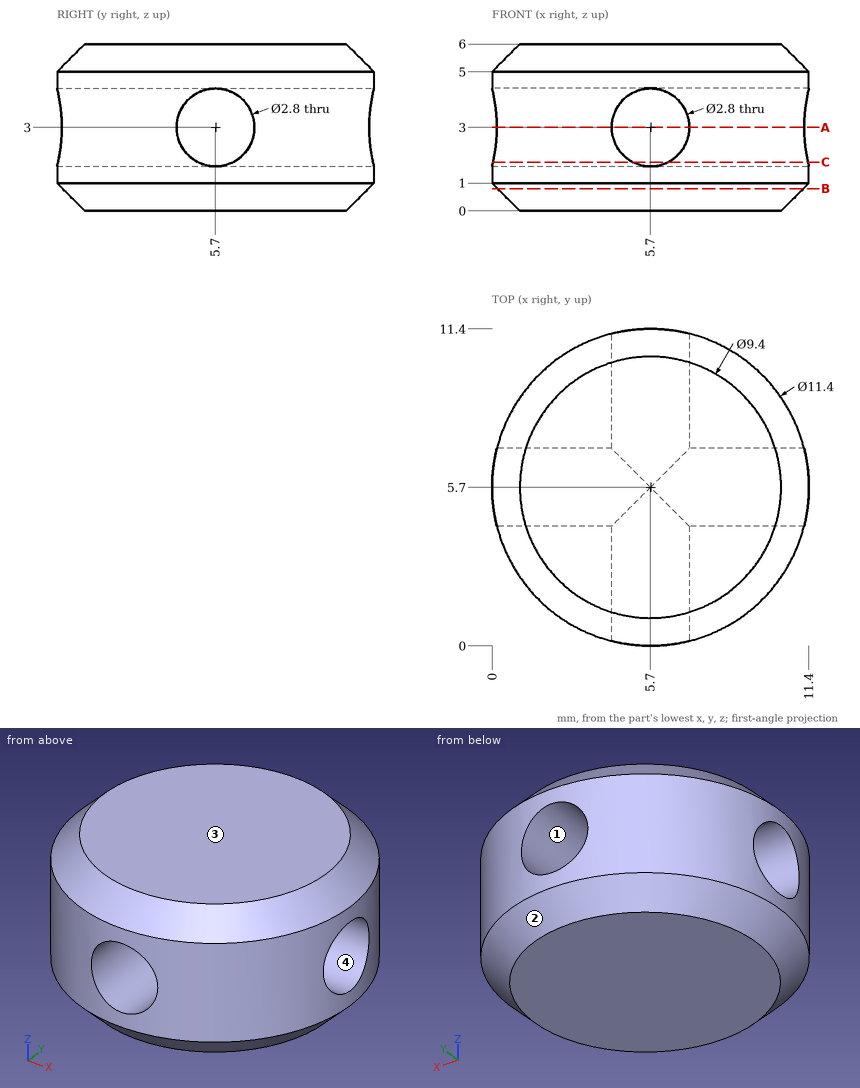
Design review of the part shown in the three views and the two pictorial views. Dimensions are in mm from the part's minimum x, y and z. Round coordinates to 2 decimals unless told otherwise and drop trailing zeros. Write each loop counter-clockwise with the first axis right and the second up, starting at its lowest first coordinate (ties: lowest second). Pieces come first, ordered by that corner, then holes.
1) Take a section at A-A on z = 3. Give the boundary of the cut face in (x, y).
Answer below:
outline: (0.17, 4.3) arc R5.7 ccw to (4.3, 0.17) - (4.3, 4.3) - close; (0.17, 7.1) - (4.3, 7.1) - (4.3, 11.23) arc R5.7 ccw to start; (7.1, 0.17) arc R5.7 ccw to (11.23, 4.3) - (7.1, 4.3) - close; (7.1, 7.1) - (11.23, 7.1) arc R5.7 ccw to (7.1, 11.23) - close
2) Insertion check: pin 1 Ø3 at (x, z) = (5.7, 3) entering from +Y; pin 2 Ø2 at (y, z) = (7, 4.5) entering from -X. Each pin has a flat end and moves straight along its axis. Give the tip position at first contact, or say it passes through.
Answer below:
pin 1: stops at y = 11.4
pin 2: stops at x = 0.01
3) For line 1 along Y through (x, z) = (2.95, 3); line 2 along Z through (x, y) = (3, 5); line 3 along X through (y, z) = (10.5, 3.15), list the stretches that pass through material, from the lowest coordinate up.
Answer below:
line 1: y = 0.71 to 4.3, 7.1 to 10.69
line 2: z = 0 to 1.79, 4.21 to 6
line 3: x = 2.63 to 4.31, 7.09 to 8.77
4) Take a section at C-C on z = 1.75. Give the boundary of the cut face in (x, y).
Answer below:
outline: (0.03, 5.07) arc R5.7 ccw to (5.07, 0.03) - (5.07, 5.07) - close; (0.03, 6.33) - (5.07, 6.33) - (5.07, 11.37) arc R5.7 ccw to start; (6.33, 0.03) arc R5.7 ccw to (11.37, 5.07) - (6.33, 5.07) - close; (6.33, 6.33) - (11.37, 6.33) arc R5.7 ccw to (6.33, 11.37) - close
5) Mouldability with a two-part tool opening along Z and no side actions: class the marked faces 1, 2, 3 and 4 as +Z half, -Z half, draft (parallel to the pull), parting line (faces both ways), or undercut.
Answer below:
face 1: undercut
face 2: -Z half
face 3: +Z half
face 4: undercut
6) Take a section at B-B on z = 0.8. Give the boundary of the cut face in (x, y), then the cut area to 3 significant figures.
Answer below:
outline: circle Ø11 at (5.7, 5.7)
area: 95.0 mm2
